Autodesk Inventor part; units mm, degrees
ref_plane "Work Plane1" through (5, 0, 0) normal (0, 0.5, 0.866) x (1, 0, 0)
ref_plane "YZ Plane" through (0, 0, 0) normal (1, 0, 0) x (0, 1, 0)
ref_plane "XZ Plane" through (0, 0, 0) normal (0, 1, 0) x (-1, 0, 0)
sketch "Sketch1" plane through (0, 0, 0) normal (0, 0, 1) x (1, 0, 0)
  line L0 (0, 0) -> (6.8333, 0)
  line L1 (10, 1.1547) -> (10, 2)
  line L2 (10, 2) -> (0, 2)
  line L3 (10, 1.1547) -> (7.5, 1.1547)
  line L4 (7.5, 1.1547) -> (6.8333, 0)
  line L5 (0, -0.4) -> (0, 2.4)
  line L6 (0, 2) -> (0, 0)
  dimension "d0" = 2.5
  dimension "d1" = 60
  dimension "d2" = 4
  dimension "d3" = 2.3094
  dimension "d5" = 10
revolve "Body" add sketch "Sketch1" angle 360 about axis through (0, 0, 0) along (1, 0, 0)
chamfer "Chamfer1" distance 0.4294 angle 60 1 edges at (10, -2, 0) measured on face at (10, 1.6877, -0.2517)
sketch "Sketch2" plane through (10, 0, 0) normal (1, 0, 0) x (0, 0, -1)
  circle A0 centre (0, 0) radius 1.1547
  line L0 (-0.5774, 1) -> (0.5774, 1)
  line L1 (0.5774, 1) -> (1.1547, 0)
  line L2 (1.1547, 0) -> (0.5774, -1)
  line L3 (0.5774, -1) -> (-0.5774, -1)
  line L4 (-0.5774, -1) -> (-1.1547, 0)
  line L5 (-1.1547, 0) -> (-0.5774, 1)
  point P0 (0, 0)
  point P1 (0, 0)
extrude "Slot" add sketch "Sketch2" against normal up to next contours L1 A0 | A0 L2 | L0 A0 | A0 L3 | L5 A0 | A0 L4
thread "Thread"
chamfer "Chamfer2" distance 0.4294 angle 60 1 edges at (0, -2, 0) measured on face at (3.0854, 1.9741, -0.3208)
ref_plane "Work Plane1" through (5, 0, 0) normal (0, 0.5, 0.866) x (1, 0, 0)
equation "\"d0\" = INTI"
equation "\"d2\" = NND"
equation "\"d3\" = 1.1547 * SW"
equation "\"d5\" = NLG"
equation "\"d7\" = -0.5 * GD1 + 0.5 * NND"
equation "\"d8\" = FAWI"
equation "\"d29\" = -0.5 * GD1 + 0.5 * NND"
equation "\"d11\" = NLG"
equation "\"d13\" = -0.5 * GD1 + 0.5 * NND"
equation "\"d14\" = FAWI"
equation "\"d30\" = -0.5 * GD1 + 0.5 * NND"
equation "\"NND\" = 4"
equation "\"NLG\" = 10"
equation "\"INTI\" = 2.5"
equation "\"FAWI\" = 60deg"
equation "\"SW\" = 2"
equation "\"GD1\" = THREADDIA - 1.2269 * PTC"
equation "\"FAWI1\" = 45deg"
equation "\"GUL\" = 0.61345 * PTC"
equation "\"SPD\" = 2"
equation "\"TOA\" = 30deg"
equation "\"THREADDIA\" = 4"
equation "\"PTC\" = 0.7"
equation "\"GAL\" = 0.61345 * PTC"
equation "\"E0\" = 1.155 * SW"
properties part number "AS 1421 - M4 x 10 Flat Point" material "Steel, Mild"
Part model, mm, in its own coordinate system. Round coordinates to 2 decimals unless told otherwise and drop trailing zeros. Loops run counter-clockwise (first coordinate to the right, second up) from the corner with the lowest first, then second, coordinate; pieces in that order, holes last.
Item 1: Drop a flat-ended pin along its axis: P1, Ø1.5, axis at x = 6, y = -1, coming from the +Z side. Give the stop position or say it passes through.
Item 2: Drill centre lines: line 1 (Y direction, x = 7.75, z = 0.65); line 2 (Y direction, x = 9.75, z = 0.05); line 3 (Z direction, x = 8.75, y = 0.65). Where is each one in solid material? Low to high.
Item 3: Cut at B-B, the plane x = 3.25. Give the cut face in (y, z), then the cut area to 3 significant figures.
Item 4: Mould opens along Z. For faces 1 (the face through (0, 0, 0)), 2 (the face through (8.72, -0.51, 0.86)), 3 (the face through (5, 0, 2)) say: +Z half, -Z half, draft (parallel to the pull), parting line (faces both ways), or undercut.
Item 5: Cut at A-A, the plane x = 8.25. Give the cut face in (y, z).
A:
1. P1: stops at z = 1.98
2. line 1: y = -1.89 to -0.87, 0.87 to 1.89
2. line 2: y = -1.71 to -1, 1 to 1.71
2. line 3: z = -1.89 to -0.78, 0.78 to 1.89
3. outline: circle Ø4 at (0, 0)
3. area: 12.6 mm2
4. face 1: draft
4. face 2: undercut
4. face 3: parting line
5. outline: circle Ø4 at (0, 0); hole (-1, -0.58) - (0, -1.15) - (1, -0.58) - (1, 0.58) - (0, 1.15) - (-1, 0.58) - close
